Solid Edge part; units mm, degrees
sketch "Sketch1" plane through (0, 0, 0) normal (0, 0, 1) x (1, 0, 0)
  line L0 (2.5, 0) -> (2.5, 40)
  line L1 (0, 40) -> (2.5, 40)
  line L2 (0, 0) -> (0, 40)
  line L3 (0, 0) -> (0, -5)
  line L4 (0, -5) -> (4.25, -5)
  line L5 (4.25, -5) -> (4.25, 0)
  line L6 (4.25, 0) -> (2.5, 0)
revolve "RevolvedProtrusion1" add sketch "Sketch1" angle 360 about axis through (0, 0, 0) along (0, 1, 0)
sketch "Sketch2" plane through (0, 0, 0) normal (1, 0, 0) x (0, 1, 0)
  line L0 (-5, 2.7915) -> (-2.5, 2.7915)
  line L1 (-0.8883, 0) -> (-2.5, 2.7915)
  line L2 (-5, 0) -> (-0.8883, 0)
  line L3 (-5, 0) -> (-5, 2.7915)
revolve "RevolvedCutout1" cut sketch "Sketch2" angle 360 about axis through (0, -4.5, 0) along (0, 1, 0)
sketch "Sketch3" plane through (0, -5, 0) normal (0, -1, 0) x (0, 0, 1)
  circle A0 centre (0, 0) radius 2.7915
  line L0 (-2, -1.1547) -> (0, -2.3094)
  line L1 (0, -2.3094) -> (2, -1.1547)
  line L2 (2, -1.1547) -> (2, 1.1547)
  line L3 (2, 1.1547) -> (0, 2.3094)
  line L4 (0, 2.3094) -> (-2, 1.1547)
  line L5 (-2, 1.1547) -> (-2, -1.1547)
extrude "Protrusion1" add sketch "Sketch3" against normal up to next
sketch "Sketch4" plane through (0, 0, 0) normal (0, 0, 1) x (1, 0, 0)
  line L0 (-2.3094, -5) -> (0, -5)
  line L1 (0, -5) -> (0, -4.3812)
  line L2 (0, -4.3812) -> (-2.3094, -5)
revolve "RevolvedCutout2" cut sketch "Sketch4" angle 360 about axis through (0, -4.5, 0) along (0, 1, 0)
fillet "Round1" radius 0.2 1 edges at (0, 0, -2.5)
fillet "Round2" radius 0.425 1 edges at (0, -5, -4.25)
chamfer "倒斜角_2" distance 0.3333 angle 45 1 edges at (0, 40, -2.5)
cosmetic_thread "螺纹_3" thread depth 32
properties part number "N2611-031G" material "铝 1060"
Design review of the part built by this model. Coordinates are the model's own, in mm. A direction names the side the tool comes from. Coordinates: 2 decimals unless noted, no trailing zeros. Order: outer loops, then holes, each group sorted by start corner. A loop starts at its lowest first (then second) coordinate and runs counter-clockwise, first axis right, second up. Notation, with made-up numbers: M 48.5,-16.5 L 53.5,-16.5 A23 cw 53.5,10.5 Z; hole C 22,65.25 d11. An arc over 180 degrees is marked long. Answer as a JSON object with one key per item and string values. Group by question number.
1) Add section A-A, the plane y = 2. Write out the cut boundary in (x, z).
2) Tool access review of faces 1 (the flat face through (2, -5, 2)), 2 (the flat face through (-1.724, -3.542, 1.014)), 3 (the cylindrical face through (-0.54, 20.21, 2.44)): name each direction out of +Z, -Z, +X, -X, +Y, -Y from which nothing blocks a thin tool from reaching the whole face with its end or side.
3) Wall thickness on L1, parallel to Y at x = -3.25, z = -0.5; L2, parallel to X at y = -2, z = 0.75; L3, parallel to Z at x = -1.5, y = 22.5: over which ranges is each line inside the solid? List them lowest first.
4) For pin 1 (1 mm diameter, centred on x = -1, y = 27, fed in from -Z); pin 2 (2 mm diameter, centred on y = 4, z = 1.5, fed in from -X), all flat-tipped, find the tip position at first contact; note any pin that passes through.
5) Mouldability with a two-part tool opening along Z and no side actions: class faces 4 (the cylindrical face through (2.285, -2.255, -3.584)), 5 (the flat face through (1.74, -3.54, 0.99)), 6 (the flat face through (0, 0, 3)) as pulls with the +Z half, pulls with the -Z half, needs draft (parallel to the pull), parting line crosses it, or undercut.
Computed values:
{
 "1": {"outline": "C 0,0 d5"},
 "2": {"face 1": "+Z, -Z, +X, -X, -Y", "face 2": "-Y", "face 3": "+Y"},
 "3": {"L1": "y = -5 to 0", "L2": "x = -4.18 to -1.77, 1.77 to 4.18", "L3": "z = -2 to 2"},
 "4": {"pin 1": "stops at z = -2.45", "pin 2": "stops at x = -2.45"},
 "5": {"face 4": "parting line crosses it", "face 5": "undercut", "face 6": "needs draft"}
}
